Source: CAD feature listing. Evaluate the final solid. Frame: model axes, mm. A direction names the side the tool comes from. Round coordinates to 2 decimals unless told otherwise and drop trailing zeros. Order: outer loops, then holes, each group sorted by start corner. A loop starts at its lowest first (then second) coordinate and runs counter-clockwise, first axis right, second up.
```python
from build123d import *

# Parameters (mm, degrees)
F0_W     = 200
F0_H     = 64.601768
F1_DEPTH = 1
F2_W     = 1
F2_H     = 64.601768
F3_DEPTH = 20
F4_W     = 199
F4_H     = 1
F5_DEPTH = 20
F6_W     = 199
F6_H     = 1
F7_DEPTH = 20
F8_W     = 1
F8_H     = 62.601768
F9_DEPTH = 20


with BuildPart() as f1:
    # F0 (on Top) → F1 (new body)
    with BuildSketch(Plane.XY):
        Rectangle(F0_W, F0_H)
    extrude(amount=F1_DEPTH)

    # F2 (on face) → F3 (join)
    with BuildSketch(Plane.XY.offset(1)):
        with Locations((-99.5, 0)):
            Rectangle(F2_W, F2_H)
    extrude(amount=F3_DEPTH)

    # F4 (on face) → F5 (join)
    with BuildSketch(Plane.XY.offset(1)):
        with Locations((0.5, 31.800884)):
            Rectangle(F4_W, F4_H)
    extrude(amount=F5_DEPTH)

    # F6 (on face) → F7 (join)
    with BuildSketch(Plane.XY.offset(1)):
        with Locations((0.5, -31.800884)):
            Rectangle(F6_W, F6_H)
    extrude(amount=F7_DEPTH)

    # F8 (on face) → F9 (join)
    with BuildSketch(Plane.XY.offset(1)):
        with Locations((99.5, 0)):
            Rectangle(F8_W, F8_H)
    extrude(amount=F9_DEPTH)


solid = f1.part
```
1. Access query for faces 4 (the face through (-99, 0, 11)), 5 (the face through (-100, 0, 10)). Directions: +Z, -Z, +X, -X, +Y, -Y. A direction counts if a zero-diameter tool reaches every point of the face in a straight line with its end or side. Return the directions, or none.
2. Section C-C on y = 11.5. Return loops of the section in (x, z), plus the area to 3 significant figures.
3. Section B-B on x = -39.5. Return loops of the section in (y, z), plus the area to 3 significant figures.
4. Line query: line 1 along Y through (x, z) = (-0.5, 2); line 2 along X through (y, z) = (3, 5.5); line 3 along Z through (x, y) = (-62, -28). Output: solid intervals per line, ascending.
5. Pull-direction query (Y, two-part tool) for faces 1 (the face through (-1, 32.301, 10)), 2 (the face through (-1, 0, 1)), 3 (the face through (-1, 0, 0)); classes: released by +Y, released by -Y, zero draft, split by the parting line, or undercut.
6. First-contact query: pin 1 (5 mm diameter, centred on x = -28, y = 5, fed in from +Z). Flat tip, straight axial feed; report the tip coordinate or a pass-through.
7. Section A-A on z = 7. Return loops of the section in (x, y).
Result:
1. face 4: +Z
1. face 5: +Z, -Z, -X, +Y, -Y
2. outline: (-100, 0) - (100, 0) - (100, 21) - (99, 21) - (99, 1) - (-99, 1) - (-99, 21) - (-100, 21) - close
2. area: 240 mm2
3. outline: (-32.3, 0) - (32.3, 0) - (32.3, 21) - (31.3, 21) - (31.3, 1) - (-31.3, 1) - (-31.3, 21) - (-32.3, 21) - close
3. area: 105 mm2
4. line 1: y = -32.3 to -31.3, 31.3 to 32.3
4. line 2: x = -100 to -99, 99 to 100
4. line 3: z = 0 to 1
5. face 1: released by +Y
5. face 2: undercut
5. face 3: zero draft
6. pin 1: stops at z = 1
7. outline: (-100, -32.3) - (100, -32.3) - (100, 32.3) - (-100, 32.3) - close; hole (-99, -31.3) - (99, -31.3) - (99, 31.3) - (-99, 31.3) - close
